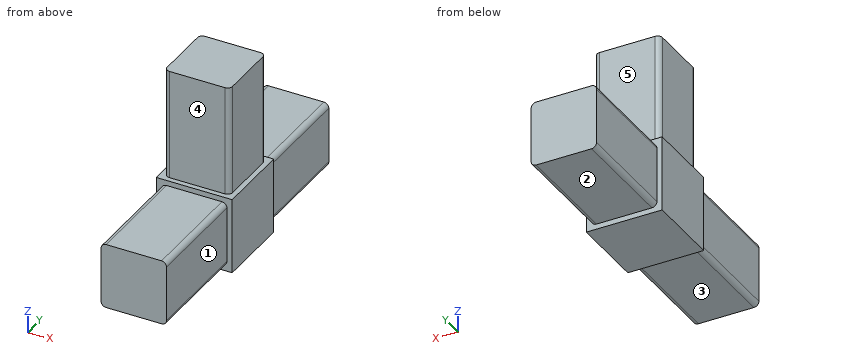
```python
from build123d import *

# Parameters (mm, degrees)
SKETCH1_W           = 16.637
SKETCH1_H           = 16.637
BOSS_EXTRUDE1_DEPTH = 28.067
SKETCH2_W           = 19.304
SKETCH2_H           = 19.304
BOSS_EXTRUDE2_DEPTH = 19.304
SKETCH3_W           = 16.637
SKETCH3_H           = 16.637
BOSS_EXTRUDE3_DEPTH = 28.067
SKETCH5_W           = 16.637
SKETCH5_H           = 16.637
BOSS_EXTRUDE4_DEPTH = 28.067
FILLET1_R           = 1.27


with BuildPart() as part:
    # Sketch1 → Boss-Extrude1 (new body)
    with BuildSketch(Plane(origin=(0, 0, 0), x_dir=(1, 0, 0), z_dir=(0, 1, 0))):
        Rectangle(SKETCH1_W, SKETCH1_H)
    extrude(amount=BOSS_EXTRUDE1_DEPTH)

    # Sketch2 → Boss-Extrude2 (add)
    with BuildSketch(Plane(origin=(0, 28.067, 0), x_dir=(1, 0, 0), z_dir=(0, 1, 0))):
        Rectangle(SKETCH2_W, SKETCH2_H)
    extrude(amount=BOSS_EXTRUDE2_DEPTH)

    # Sketch3 → Boss-Extrude3 (add)
    with BuildSketch(Plane.XY.offset(9.652)):
        with Locations((0, 37.719)):
            Rectangle(SKETCH3_W, SKETCH3_H)
    extrude(amount=BOSS_EXTRUDE3_DEPTH)

    # Sketch5 → Boss-Extrude4 (add)
    with BuildSketch(Plane(origin=(0, 47.371, 0), x_dir=(1, 0, 0), z_dir=(0, 1, 0))):
        Rectangle(SKETCH5_W, SKETCH5_H)
    extrude(amount=BOSS_EXTRUDE4_DEPTH)

    # Fillet1
    fillet1_edges = [part.edges().sort_by_distance(p)[0] for p in [
        (8.3185, 29.4005, 23.6855),
        (8.3185, 46.0375, 23.6855),
        (-8.3185, 46.0375, 23.6855),
        (-8.3185, 29.4005, 23.6855),
        (8.3185, 61.4045, 8.3185),
        (8.3185, 61.4045, -8.3185),
        (-8.3185, 61.4045, -8.3185),
        (-8.3185, 61.4045, 8.3185),
        (8.3185, 14.0335, 8.3185),
        (-8.3185, 14.0335, 8.3185),
        (-8.3185, 14.0335, -8.3185),
        (8.3185, 14.0335, -8.3185),
    ]]
    fillet(fillet1_edges, radius=FILLET1_R)


solid = part.part
```
Check sheet for the modelled part. Datum: model origin and axes. Units: mm. Face numbers are marked on the shaded views. A direction names the side the tool comes from. Round coordinates to 2 decimals unless told otherwise and drop trailing zeros. Loops run counter-clockwise (first coordinate to the right, second up) from the corner with the lowest first, then second, coordinate; pieces in that order, holes last. Notation, with made-up numbers: (48, 40.5) - (74, 40.5) arc R15 ccw to (74, 63.5) - close; hole circle Ø4 at (44, 53.5). An arc over 180 degrees is marked (long way). Answer as a JSON object with one key per item and string values. Group by question number.
Q1. Sectioned sample at D-D, the plane z = -1. Enter the section's corners in (x, y), plus the area to 3 significant figures.
Q2. Scan lines: line 1 along X through (y, z) = (28, 7); line 2 along Y through (x, z) = (6.75, 21). Record each from-to range of solid material in increasing order. Write a range as [from, to].
Q3. Set-up check for the marked faces 1, 2, 3, 4 and 5: record each of +Z, -Z, +X, -X, +Y, -Y from which the full face is reachable in a straight line by a thin tool's end or side.
Q4. Gauge pin test, flat ends, axial feed: P1, Ø5, axis at x = 5, y = 58, coming from the -Z side; P2, Ø7, axis at y = 36.5, z = 23.5, coming from the +X side; P3, Ø4, axis at x = -2, z = 20.5, coming from the +Y side. Record the tip position at first contact, or that the pin passes through.
Q5. Sectioned sample at B-B, the plane z = 32. Enter the section's corners in (x, y), plus the area to 3 significant figures.
Q6. Sectioned sample at A-A, the plane x = 0.5. Enter the section's corners in (y, z), plus the area to 3 significant figures.
Q7. Sectioned sample at C-C, the plane y = 42.5. Enter the section's corners in (x, z).
Solution:
{
 "1": {"outline": "(-9.65, 28.07) - (-8.32, 28.07) - (-8.32, 0) - (8.32, 0) - (8.32, 28.07) - (9.65, 28.07) - (9.65, 47.37) - (8.32, 47.37) - (8.32, 75.44) - (-8.32, 75.44) - (-8.32, 47.37) - (-9.65, 47.37) - close", "area": "1,310 mm²"},
 "2": {"line 1": "x = [-8.32, 8.32]", "line 2": "y = [29.4, 46.04]"},
 "3": {"face 1": "+Z, -Z, +X, -Y", "face 2": "-Z, +X, -X, +Y", "face 3": "-Z, +X, -X, -Y", "face 4": "+Z, +X, -X, -Y", "face 5": "+Z, +X, -X, +Y"},
 "4": {"P1": "stops at z = -8.32", "P2": "stops at x = 8.32", "P3": "stops at y = 46.04"},
 "5": {"outline": "(-8.32, 30.67) arc R1.27 ccw to (-7.05, 29.4) - (7.05, 29.4) arc R1.27 ccw to (8.32, 30.67) - (8.32, 44.77) arc R1.27 ccw to (7.05, 46.04) - (-7.05, 46.04) arc R1.27 ccw to (-8.32, 44.77) - close", "area": "275 mm²"},
 "6": {"outline": "(0, -8.32) - (28.07, -8.32) - (28.07, -9.65) - (47.37, -9.65) - (47.37, -8.32) - (75.44, -8.32) - (75.44, 8.32) - (47.37, 8.32) - (47.37, 9.65) - (46.04, 9.65) - (46.04, 37.72) - (29.4, 37.72) - (29.4, 9.65) - (28.07, 9.65) - (28.07, 8.32) - (0, 8.32) - close", "area": "1,770 mm²"},
 "7": {"outline": "(-9.65, -9.65) - (9.65, -9.65) - (9.65, 9.65) - (8.32, 9.65) - (8.32, 37.72) - (-8.32, 37.72) - (-8.32, 9.65) - (-9.65, 9.65) - close"}
}
